from build123d import *

# Parameters (mm, degrees)
SKETCH2_W               = 50.634745493
SKETCH2_H               = 13.07277583
CUT_EXTRUDE1_DEPTH      = 5.0000001
CUT_EXTRUDE1_DEPTH_BACK = 5.0000001
SKETCH3_R               = 1
CUT_EXTRUDE2_DEPTH      = 5.0000001
SKETCH4_R               = 2.1
CUT_EXTRUDE3_DEPTH      = 4.0000001
SKETCH5_R               = 1.5
CUT_EXTRUDE4_DEPTH      = 5.0000001


with BuildPart() as part:
    # Sketch1 → Revolve1 (revolve)
    with BuildSketch(Plane.XY):
        with BuildLine():
            Line((-14, 0), (14, 0))
            add(Edge.make_bspline(
                [(14, 0), (14, 4), (0, 4), (-14, 4), (-14, 0)],
                knots=[0, 0, 0, 1.570796327, 1.570796327, 3.141592654, 3.141592654, 3.141592654], degree=2, weights=[1, 0.707106781, 1, 0.707106781, 1]))
        make_face()
    revolve(axis=Axis((-14, 0, 0), (1, 0, 0)))

    # Sketch2 → Cut-Extrude1 (cut, two sides)
    with BuildSketch(Plane.XY) as cut_extrude1_sk:
        with Locations((-1.598405816, -6.536387915)):
            Rectangle(SKETCH2_W, SKETCH2_H)
    extrude(amount=CUT_EXTRUDE1_DEPTH, mode=Mode.SUBTRACT)
    extrude(cut_extrude1_sk.sketch, amount=-CUT_EXTRUDE1_DEPTH_BACK, mode=Mode.SUBTRACT)

    # Sketch3 → Cut-Extrude2 (cut, through all)
    with BuildSketch(Plane.XZ):
        with Locations((-10.5, 0)):
            Circle(SKETCH3_R)
        with Locations((10.5, 0)):
            Circle(SKETCH3_R)
    extrude(amount=-CUT_EXTRUDE2_DEPTH, mode=Mode.SUBTRACT)

    # Sketch4 → Cut-Extrude3 (cut, through all)
    with BuildSketch(Plane(origin=(0, 1, 0), x_dir=(-1, 0, 0), z_dir=(0, -1, 0))):
        with Locations((10.5, 0)):
            Circle(SKETCH4_R)
        with Locations((-10.5, 0)):
            Circle(SKETCH4_R)
    extrude(amount=-CUT_EXTRUDE3_DEPTH, mode=Mode.SUBTRACT)

    # Sketch5 → Cut-Extrude4 (cut, through all)
    with BuildSketch(Plane.XZ):
        with Locations((-4.5, 2)):
            Circle(SKETCH5_R)
        with Locations((-4.5, -2)):
            Circle(SKETCH5_R)
    extrude(amount=-CUT_EXTRUDE4_DEPTH, mode=Mode.SUBTRACT)


solid = part.part
The listing builds one solid part. Answer for the finished solid, in the listing's coordinates (mm). A direction names the side the tool comes from. Round coordinates to 2 decimals unless told otherwise and drop trailing zeros. Write each question's results on one line, items separated by ' | '. Start each with the question number.
Q1. Each of these flat-tipped pins is pushed along its axis until it touches: pin 1 (1.6 mm diameter, centred on x = -10.5, z = 0, fed in from -Y); pin 2 (2 mm diameter, centred on y = 1, z = -1.5, fed in from -X); pin 3 (3.5 mm diameter, centred on x = 10, z = -0.5, fed in from +Y); pin 4 (2 mm diameter, centred on x = -10, z = 1.5, fed in from -Y). Where does it stop, or does it pass through?
Q2. Find section A-A (x = -4.5). Give the number of separate pieces and of enclosed holes in the cut face, then the cut area to 3 significant figures.
Q3. Which of the six approach directions +Z, -Z, +X, -X, +Y, -Y give full straight-line access (tool end or side, diameter ignored) to faces 1 (the cylindrical face through (8.497, 1.596, -0.631)), 2 (the flat face through (0, 0, 0))?
Q4. Straight lines are drawn through the part: probe 1 along X at (y, z) = (0.6, 0.25); probe 2 along Z at (x, y) = (-4.25, 0.9); probe 3 along Y at (x, z) = (-11.5, 0.75). For each, find the intervals that lie inside material, in ascending order. Write a range as from..to.
Worked answers:
1) pin 1: passes through | pin 2: stops at x = -13.72 | pin 3: stops at y = 3.22 | pin 4: stops at y = 0
2) separate pieces: 3 | enclosed holes: 0 | area: 4.34 mm2
3) face 1: +Y | face 2: +Z, -Z, +X, -X, -Y
4) probe 1: x = -13.81..-11.47, -9.53..9.53, 11.47..13.81 | probe 2: z = -3.7..-3.48, -0.52..0.52, 3.48..3.7 | probe 3: y = 0..1
